Geometry: final body of the model. Coordinates: model frame, mm. A direction names the side the tool comes from. Coordinates: 2 decimals unless noted, no trailing zeros. Write each loop counter-clockwise with the first axis right and the second up, starting at its lowest first coordinate (ties: lowest second). Pieces come first, ordered by that corner, then holes. Notation, with made-up numbers: M -21.5,-21 L -8.5,-21 A20 ccw -8.5,-15 Z; hole C 79.5,-23.5 d3. An arc over 180 degrees is marked long. Write item = value, one per line. Start each with the question number.
Item 1: Reachability of faces 1 (the flat face through (52, 22, 15)), 2 (the flat face through (53, 19, 14.75)), 3 (the flat face through (49.5, 21.8, 5.6)) from +Z, -Z, +X, -X, +Y, -Y: full face, straight path, thin tool, end or side. Return the list, or none.
Item 2: First-contact query: pin 1 Ø1.2 at (x, z) = (3, 15.25) entering from -Y; pin 2 Ø6 at (x, z) = (27.5, 10.5) entering from +Y; pin 3 Ø1.6 at (x, z) = (52.5, 15.25) entering from +Y. Flat tips, straight axial feed; report the tip coordinate or a pass-through.
Item 3: Section C-C on y = 5. Output: boundary loops of the cut face in (x, z).
Item 4: Section B-B on x = 3. Output: boundary loops of the cut face in (y, z).
Item 5: Section A-A on y = 17.5. Output: boundary loops of the cut face in (x, z), plus the area to 3 significant figures.
Item 6: Ray query, L1, parallel to Z at x = 3, y = 8; L2, parallel to X at y = 26.25, z = 15.25; L3, parallel to X at y = 11, z = 15.25. Return the intervals inside material, ascending. Write a range as [from, to].
Item 7: Pull-direction query (X, two-part tool) for faces 4 (the flat face through (6, 22, 10)), 5 (the flat face through (55.5, 18.7, 5.6)), 6 (the flat face through (3, 38, 10)); classes: +X half, -X half, draft (parallel to the pull), parting line (faces both ways), or undercut.
Item 8: Section D-D on x = 37.5. Output: boundary loops of the cut face in (y, z), plus the area to 3 significant figures.
Autodesk Inventor part; units mm, degrees
ref_plane "YZ Plane" through (0, 0, 0) normal (1, 0, 0) x (0, 1, 0)
ref_plane "XZ Plane" through (0, 0, 0) normal (0, 1, 0) x (-1, 0, 0)
ref_plane "XY Plane" through (0, 0, 0) normal (0, 0, 1) x (1, 0, 0)
sketch "Эскиз1" plane through (0, 0, 0) normal (0, 0, 1) x (1, 0, 0)
  line L0 (0, 0) -> (55.5, 0)
  line L1 (55.5, 0) -> (55.5, 6)
  line L2 (55.5, 6) -> (0, 6)
  line L3 (0, 6) -> (0, 0)
  line L4 (0, 6) -> (6, 6)
  line L5 (6, 6) -> (6, 38)
  line L6 (6, 38) -> (0, 38)
  line L7 (0, 38) -> (0, 6)
  line L8 (55.5, 6) -> (49.5, 6)
  line L9 (49.5, 6) -> (49.5, 38)
  line L10 (49.5, 38) -> (55.5, 38)
  line L11 (55.5, 38) -> (55.5, 6)
  dimension "d0" = 38
  dimension "d1" = 6
  dimension "d2" = 6
  dimension "d3" = 6
  dimension "d4" = 38
  dimension "d5" = 55.5
extrude "Выдавливание1" add sketch "Эскиз1" along normal blind 20.5
sketch "Эскиз2" plane through (55.5, 0, 0) normal (1, 0, 0) x (0, 0, -1)
  circle A0 centre (-10.25, 26.5) radius 4.5
  circle A1 centre (-10.25, 11.5) radius 4.5
  line L0 (-5.75, 26.5) -> (-5.75, 11.5)
  line L1 (-14.75, 26.5) -> (-14.75, 11.5)
  line L2 (0, 0) -> (-20.5, 0)
  point P0 (-10.25, 0)
  dimension "d8" = 9
  dimension "d9" = 11.5
  dimension "d10" = 24
extrude "Выдавливание2" cut sketch "Эскиз2" against normal up to next
sketch "Эскиз3" plane through (0, 0, 0) normal (0, -1, 0) x (1, 0, 0)
  circle A0 centre (37.5, 10.25) radius 2
  line L0 (55.5, 0) -> (55.5, 20.5)
  point P0 (0, 0)
  point P1 (55.5, 10.25)
  dimension "d13" = 4
  dimension "d14" = 18
extrude "Выдавливание3" cut sketch "Эскиз3" against normal up to next
sketch "Эскиз4" plane through (49.5, 38, 0) normal (0, 1, 0) x (1, 0, 0)
  circle A0 centre (3, -15.25) radius 1
  circle A1 centre (3, -5.25) radius 1
  line L0 (0, 0) -> (0, -20.5)
  line L1 (6, -20.5) -> (0, -20.5)
  line L2 (3, -5.25) -> (3, -15.25) construction
  point P0 (-49.5, 0)
  point P1 (3, -10.25)
  point P2 (0, -10.25)
  dimension "d17" = 2
  dimension "d18" = 10
  dimension "d19" = 2
extrude "Выдавливание4" cut sketch "Эскиз4" against normal blind 16
sketch "Эскиз5" plane through (0, 38, 0) normal (0, 1, 0) x (1, 0, 0)
  circle A0 centre (3, -5.25) radius 1
  circle A1 centre (3, -15.25) radius 1
  circle A2 centre (52.5, -5.25) radius 1
  circle A3 centre (52.5, -15.25) radius 1
  line L0 (6, 0) -> (0, 0)
  point P0 (3, 0)
  dimension "d23" = 2
extrude "Выдавливание5" cut sketch "Эскиз5" against normal up to next contours A0 | A1
sketch "Эскиз6" plane through (0, 0, 20.5) normal (0, 0, 1) x (1, 0, 0)
  point P0 (0, 0)
properties part number "kreplenie2"
Responses:
q1.face_1 = +Y
q1.face_2 = +X
q1.face_3 = +Z, -Z, +Y
q2.pin_1 = through
q2.pin_2 = 6
q2.pin_3 = 22
q3.outline = M 0,0 L 55.5,0 L 55.5,20.5 L 0,20.5 Z; hole C 3,5.25 d2; hole C 3,15.25 d2; hole C 37.5,10.25 d4
q4.outline = M 0,0 L 38,0 L 38,4.25 L 0,4.25 Z; M 0,6.25 L 38,6.25 L 38,14.25 L 0,14.25 Z; M 0,16.25 L 38,16.25 L 38,20.5 L 0,20.5 Z
q5.outline = M 0,0 L 6,0 L 6,20.5 L 0,20.5 Z; M 49.5,0 L 55.5,0 L 55.5,5.75 L 49.5,5.75 Z; M 49.5,14.75 L 55.5,14.75 L 55.5,20.5 L 49.5,20.5 Z; hole C 3,5.25 d2; hole C 3,15.25 d2
q5.area = 186 mm²
q6.L1 = [0, 4.25], [6.25, 14.25], [16.25, 20.5]
q6.L2 = [0, 2], [4, 6], [49.5, 51.5], [53.5, 55.5]
q6.L3 = [0, 2], [4, 6], [49.5, 55.5]
q7.face_4 = undercut
q7.face_5 = +X half
q7.face_6 = draft
q8.outline = M 0,0 L 6,0 L 6,8.25 L 0,8.25 Z; M 0,12.25 L 6,12.25 L 6,20.5 L 0,20.5 Z
q8.area = 99.0 mm²
